Build history of the part. All positions in model axes, mm. A direction names the side the tool comes from. Round coordinates to 2 decimals unless told otherwise and drop trailing zeros. Loops run counter-clockwise (first coordinate to the right, second up) from the corner with the lowest first, then second, coordinate; pieces in that order, holes last. Notation, with made-up numbers: M -13.5,-9 L -4.5,-9 A25 cw -4.5,13 Z; hole C 54,1.5 d2. An arc over 180 degrees is marked long. One line per item, written item: value.
```python
from build123d import *

# Parameters (mm, degrees)
BOSS_EXTRUDE2_DEPTH     = 6.5
SKETCH4_R               = 8
BOSS_EXTRUDE3_DEPTH     = 2
CUT_EXTRUDE1_DEPTH      = 7.37
CUT_EXTRUDE1_DEPTH_BACK = 2.37
SKETCH1_W               = 6.43
SKETCH1_H               = 6.43
FILLET1_R               = 0.5
FILLET2_R               = 0.5


with BuildPart() as part:
    # Sketch3 → Boss-Extrude2 (new body)
    with BuildSketch(Plane(origin=(0, 0, 0), x_dir=(1, 0, 0), z_dir=(0, 1, 0))):
        Polygon((2.765507789, -0.261150073), (5.531015579, 4.528849927), (2.765507789, 9.318849927), (-2.765507789, 9.318849927), (-5.531015579, 4.528849927), (-2.765507789, -0.261150073), align=None)
    extrude(amount=BOSS_EXTRUDE2_DEPTH)

    # Sketch4 → Boss-Extrude3 (add)
    with BuildSketch(Plane(origin=(0, 0, 0), x_dir=(1, 0, 0), z_dir=(0, 1, 0))):
        with Locations(Location((0, 4.528849927, 0), (0, 0, 270))):
            Circle(SKETCH4_R)
    extrude(amount=-BOSS_EXTRUDE3_DEPTH)

    # Sketch1 → Cut-Extrude1 (cut, two sides: drawn at the far end of the back side and taken through both)
    with BuildSketch(Plane(origin=(0, 0, 0), x_dir=(1, 0, 0), z_dir=(0, 1, 0)).offset(-CUT_EXTRUDE1_DEPTH_BACK)):
        with Locations((0.005, 4.528849927)):
            Rectangle(SKETCH1_W, SKETCH1_H)
    extrude(amount=CUT_EXTRUDE1_DEPTH + CUT_EXTRUDE1_DEPTH_BACK, mode=Mode.SUBTRACT)

    # Fillet1
    fillet1_edges = [part.edges().sort_by_distance(p)[0] for p in [
        (3.22, 2.25, -7.743849927),
        (-3.21, 2.25, -7.743849927),
        (-3.21, 2.25, -1.313849927),
        (3.22, 2.25, -1.313849927),
    ]]
    fillet(fillet1_edges, radius=FILLET1_R)

    # Fillet2
    fillet2_edges = [part.edges().sort_by_distance(p)[0] for p in [
        (-2.765507789, 3.25, 0.261150073),
        (-5.531015579, 3.25, -4.528849927),
        (-2.765507789, 3.25, -9.318849927),
        (2.765507789, 3.25, -9.318849927),
        (5.531015579, 3.25, -4.528849927),
        (2.765507789, 3.25, 0.261150073),
    ]]
    fillet(fillet2_edges, radius=FILLET2_R)


solid = part.part
```
Item 1: Slice it at C-C, the plane z = -6. Give the cut face in (x, y).
Check values:
outline: M -7.86,-2 L -3.21,-2 L -3.21,6.5 L -4.68,6.5 L -4.68,0 L -7.86,0 Z; M 3.22,-2 L 7.86,-2 L 7.86,0 L 4.68,0 L 4.68,6.5 L 3.22,6.5 Z
Item 2: Which spindle directions (+Z, -Z, +X, -X, +Y, -Y) get a long thin tool onto all of the face, cutting with end or side? Do faces 4 (the face through (4.17, 3.2, -6.89)), 5 (the face through (-4.166, 3.204, -2.164)), 6 (the face through (4.13, 3.2, -2.1)), 7 (the face through (0, 2, -1.314)). Say none if no direction does.
Check values:
face 4: -Z, +X, +Y
face 5: +Z, -X, +Y
face 6: +Z, +X, +Y
face 7: +Y, -Y
Item 3: Slice it at D-D, the plane x = 3.75. Give the cut face in (y, z), and give its area (3 significant figures).
Check values:
outline: M -2,-11.6 L 0,-11.6 L 0,-7.61 L 6.5,-7.61 L 6.5,-1.44 L 0,-1.44 L 0,2.54 L -2,2.54 Z
area: 68.4 mm2
Item 4: Drop flat-ended pins along their axis: P1, Ø5, axis at y = 5, z = -5.5, coming from the +X side; P2, Ø1, axis at y = 2, z = -5.5, coming from the +X side; P3, Ø5, axis at y = 4.5, z = -1, coming from the +X side. Give the stop position or say it passes through.
Check values:
P1: stops at x = 5.45
P2: stops at x = 5.26
P3: stops at x = 4.94
Item 5: Slice it at A-A, the plane x = 0. Give the cut face in (y, z), and give its area (3 significant figures).
Check values:
outline: M -2,-12.53 L 0,-12.53 L 0,-9.32 L 6.5,-9.32 L 6.5,-7.74 L -2,-7.74 Z; M -2,-1.31 L 6.5,-1.31 L 6.5,0.26 L 0,0.26 L 0,3.47 L -2,3.47 Z
area: 39.6 mm2
Item 6: Wall check: line 1 along Z through (x, y) = (-0.5, 4.5); line 2 along Y through (x, z) = (-6.5, -8.75); line 3 along X through (y, z) = (5.5, -6.5). Give the ranges that are in metal, low to high.
Check values:
line 1: z = -9.32 to -7.74, -1.31 to 0.26
line 2: y = -2 to 0
line 3: x = -4.39 to -3.21, 3.22 to 4.39
Item 7: Pull direction X, two halves, no side cores. Call faces 1 (the face through (3.22, 2, -4)), 2 (the face through (-4.131, 3.204, -6.954)), 3 (the face through (0, 3, 0.261)): pulls with the +X half, pulls with the -X half, needs draft (parallel to the pull), parting line crosses it, or undercut.
Check values:
face 1: undercut
face 2: pulls with the -X half
face 3: needs draft
Item 8: Slice it at B-B, the plane y = -0.25. Give the cut face in (x, z).
Check values:
outline: C 0,-4.53 d16; hole M -3.21,-7.24 A0.5 ccw -2.71,-7.74 L 2.72,-7.74 A0.5 ccw 3.22,-7.24 L 3.22,-1.81 A0.5 ccw 2.72,-1.31 L -2.71,-1.31 A0.5 ccw -3.21,-1.81 Z
